from build123d import *

# Parameters (mm, degrees)
SKETCH_1_W      = 7.47
SKETCH_1_H      = 54
EXTRUDE_1_DEPTH = 2
FILLET_1_R      = 15
FILLET_2_R      = 15


with BuildPart() as part:
    # Эскиз1 → Бобышка-Вытянуть1 (new body)
    with BuildSketch(Plane(origin=(0, 0, 0), x_dir=(1, 0, 0), z_dir=(0, 1, 0))):
        Rectangle(SKETCH_1_W, SKETCH_1_H)
    extrude(amount=EXTRUDE_1_DEPTH)

    # Скругление1
    # the kernel refuses this fillet: 15 mm, written as the material it takes off along each edge
    with BuildSketch(Plane(origin=(22.443286934, 2, 27), x_dir=(0, -1, 0), z_dir=(-1, 0, 0))) as fillet_1_piece_1:
        with BuildLine():
            CenterArc((15, -7.483314774), FILLET_1_R, 150.073565133, 29.926434867)
            Line((0, -7.483314774), (-0.3, -7.483314774))
            Line((-0.3, -7.483314774), (-0.3, 0))
            Line((-0.3, 0), (0, 0.3))
            ThreePointArc((0, 0.3), (1, 0.3), (1.74, 0.149666295))
            Line((1.74, 0.149666295), (2, 0))
        make_face()
    extrude(amount=44.886573868, mode=Mode.SUBTRACT)

    # Скругление2
    # the kernel refuses this fillet: 15 mm, written as the material it takes off along each edge
    with BuildSketch(Plane(origin=(-22.443286934, 2, -27), x_dir=(0, -1, 0), z_dir=(1, 0, 0))) as fillet_2_piece_1:
        with BuildLine():
            CenterArc((15, -7.483314774), FILLET_2_R, 150.073565133, 29.926434867)
            Line((0, -7.483314774), (-0.3, -7.483314774))
            Line((-0.3, -7.483314774), (-0.3, 0))
            Line((-0.3, 0), (0, 0.3))
            ThreePointArc((0, 0.3), (1, 0.3), (1.74, 0.149666295))
            Line((1.74, 0.149666295), (2, 0))
        make_face()
    extrude(amount=44.886573868, mode=Mode.SUBTRACT)


solid = part.part
Here's how the part is built. I have some questions about the finished solid (model axes, mm). Give positions to 0.01 mm unless a question says otherwise; leave off trailing zeros. Write each loop counter-clockwise with the first axis right and the second up, starting at its lowest first coordinate (ties: lowest second). Pieces come first, ordered by that corner, then holes. Notation, with made-up numbers: (47.5, 17) -> (59.5, 17) arc R30 ccw to (59.5, 48) -> close; hole circle Ø7 at (58, 4.25). An arc over 180 degrees is marked (long way). Use one line per item in the form item = value. Start each with the question number.
1. If I drill on L1, parallel to Y at x = -1.25, z = -24; L2, parallel to Z at x = 1.75, y = 0.7; L3, parallel to Z at x = -2, y = 0.1, over which ranges is the centre line in solid material (lowest first)?
2. Imagine slicing it at B-B on z = -21. List the corners of the cut face in (x, y) for me (3 decimals), plus the area to 3 significant figures.
3. Imagine slicing it at A-A on x = -0.5. List the corners of the cut face in (y, z) for me, plus the area to 3 significant figures.
Entries:
q1.L1 = 0 to 1.31
q1.L2 = -25.62 to 25.62
q1.L3 = -26.82 to 26.82
q2.outline = (-3.735, 0) -> (3.735, 0) -> (3.735, 1.926) -> (-3.735, 1.926) -> close
q2.area = 14.4 mm²
q3.outline = (0, -27) arc R15 ccw to (2, -19.52) -> (2, 19.52) arc R15 ccw to (0, 27) -> close
q3.area = 98.3 mm²
